Autodesk Fusion 360 part; units mm, degrees
sketch "Sketch2" plane through (0, 0, 0) normal (0, 1, 0) x (1, 0, 0)
  line L0 (76.2, 108.5) -> (-76.2, 108.5)
  line L1 (-76.2, 108.5) -> (-76.2, -108.5)
  line L2 (-76.2, -108.5) -> (76.2, -108.5)
  line L3 (76.2, -108.5) -> (76.2, 108.5)
  line L4 (76.2, 108.5) -> (-76.2, -108.5) construction
  line L5 (-76.2, 108.5) -> (76.2, -108.5) construction
  dimension "d14" = 152.4
  dimension "d15" = 217
extrude "Extrude1" add sketch "Sketch2" against normal blind 3
sketch "Sketch1" plane through (0, 0, 0) normal (0, 1, 0) x (1, 0, 0)
  line L0 (-73.2, -108.5) -> (-76.2, -108.5)
  line L1 (-76.2, -108.5) -> (-76.2, 108.5)
  line L2 (-76.2, 108.5) -> (-73.2, 108.5)
  line L3 (-73.2, 108.5) -> (-73.2, -108.5)
  line L4 (-73.2, -108.5) -> (-76.2, 108.5) construction
  line L5 (-76.2, -108.5) -> (-73.2, 108.5) construction
  line L6 (0, 0) -> (195.5563, 0) construction
  line L7 (73.2, 108.5) -> (76.2, 108.5)
  line L8 (76.2, 108.5) -> (76.2, -108.5)
  line L9 (76.2, -108.5) -> (73.2, -108.5)
  line L10 (73.2, -108.5) -> (73.2, 108.5)
  line L11 (-73.2, 108.5) -> (73.2, 108.5)
  line L12 (73.2, 108.5) -> (73.2, 105.5)
  line L13 (73.2, 105.5) -> (-73.2, 105.5)
  line L14 (-73.2, 105.5) -> (-73.2, 108.5)
  line L15 (73.2, 81.7222) -> (-73.2, 81.7222)
  line L16 (-73.2, 84.7222) -> (73.2, 84.7222)
  line L17 (73.2, 57.9444) -> (-73.2, 57.9444)
  line L18 (-73.2, 60.9444) -> (73.2, 60.9444)
  line L19 (73.2, 34.1667) -> (-73.2, 34.1667)
  line L20 (-73.2, 37.1667) -> (73.2, 37.1667)
  line L21 (73.2, 10.3889) -> (-73.2, 10.3889)
  line L22 (-73.2, 13.3889) -> (73.2, 13.3889)
  line L23 (73.2, -13.3889) -> (-73.2, -13.3889)
  line L24 (-73.2, -10.3889) -> (73.2, -10.3889)
  line L25 (73.2, -37.1667) -> (-73.2, -37.1667)
  line L26 (-73.2, -34.1667) -> (73.2, -34.1667)
  line L27 (73.2, -60.9444) -> (-73.2, -60.9444)
  line L28 (-73.2, -57.9444) -> (73.2, -57.9444)
  line L29 (73.2, -84.7222) -> (-73.2, -84.7222)
  line L30 (-73.2, -81.7222) -> (73.2, -81.7222)
  line L31 (73.2, -108.5) -> (-73.2, -108.5)
  line L32 (-73.2, -105.5) -> (73.2, -105.5)
  point P0 (-74.7, 0)
  dimension "d1" = 217
  dimension "d6" = 3
  dimension "d8" = 152.4
  dimension "d9" = 3
  dimension "d12" = 0
  dimension "d21" = 76.2
extrude "Extrude2" add sketch "Sketch1" along normal blind 42 contours L0 L1 L2 L3 L14 | L7 L8 L9 L10 L12 | L3 L10 L29 L30 | L3 L10 L27 L28 | L3 L10 L15 L16 | L3 L10 L25 L26 | L3 L10 L17 L18 | L3 L10 L23 L24 | L3 L10 L19 L20 | L3 L10 L21 L22
extrude "Extrude3" add sketch "Sketch1" along normal blind 45 contours L3 L10 L31 L32 | L3 L10 L11 L12 L13 L14
chamfer "Chamfer1" distance 1 angle 45 4 edges at (0, -3, -108.5) (-76.2, -3, 0) (76.2, -3, 0) (0, -3, 108.5) measured on face at (-25.4, -3, -36.1667) measured on face at (-25.4, -3, -36.1667) measured on face at (-25.4, -3, -36.1667) measured on face at (-25.4, -3, -36.1667)
equation "d1 = Length"
equation "Length = 217 mm"
equation "Width = 6 in"
equation "Wall_Thickness = 3 mm"
equation "d6 = Wall_Thickness"
equation "d8 = Width"
equation "d9 = Wall_Thickness"
equation "d14 = Width"
equation "d15 = Length"
equation "Height = 45 mm"
equation "d19 = Height - Wall_Thickness"
equation "d21 = Width / 2"
equation "BaseWallThickness_1 = 3 mm"
equation "BearingHolderHeight_1 = 20 mm"
equation "BearingHolderDistance_1 = 80 mm"
equation "BearingHolderDiameter_1 = 7.8 mm"
equation "BaseInsideWidth_1 = 70 mm"
equation "BaseLength_1 = 190 mm"
equation "BaseWallHeight_1 = 100 mm"
equation "d22 = Height"
equation "BaseWallThickness_2 = 3 mm"
equation "BearingHolderHeight_2 = 20 mm"
equation "BearingHolderDistance_2 = 80 mm"
equation "BearingHolderDiameter_2 = 7.8 mm"
equation "BaseInsideWidth_2 = 70 mm"
equation "BaseLength_2 = 190 mm"
equation "BaseWallHeight_2 = 100 mm"
Here's how the part is built. I have some questions about the finished solid (model axes, mm). Coordinates: 2 decimals unless noted, no trailing zeros. Loops run counter-clockwise (first coordinate to the right, second up) from the corner with the lowest first, then second, coordinate; pieces in that order, holes last. Notation, with made-up numbers: (-12, -7) - (7, -7) arc R10 cw to (7, 2) - close; hole circle Ø5 at (81.5, -1.5). An arc over 180 degrees is marked (long way). Answer as CSV lines item,"result".
Q1. If I drill on L1, parallel to X at y = 28, z = 69.5; L2, parallel to Y at x = -19, z = -26; L3, parallel to Y at x = -51.5, z = -36.5, over which ranges is the centre line in solid material (lowest first)? Write a range as [from, to].
Response:
L1,"[-76.2, -73.2], [73.2, 76.2]"
L2,"[-3, 0]"
L3,"[-3, 42]"
Q2. If we section it at A-A, the plane z = -40: Write out the boundary of the cut face in (x, y).
Response:
outline,"(-76.2, -2) - (-75.2, -3) - (75.2, -3) - (76.2, -2) - (76.2, 42) - (73.2, 42) - (73.2, 0) - (-73.2, 0) - (-73.2, 42) - (-76.2, 42) - close"
Q3. We'd pull the mould along Z, two halves only. Please class faces 1 (the face through (-73.2, 21, -71)), 2 (the face through (1, 21, 84.722)): pulls with the +Z half, pulls with the -Z half, needs draft (parallel to the pull), parting line crosses it, or undercut.
Response:
face 1,"undercut"
face 2,"undercut"
Q4. If we section it at B-B, the plane y = 9: Give the number of separate pieces and of enclosed holes in the cut face, and give its area (3 significant figures).
Response:
separate pieces,"1"
enclosed holes,"9"
area,"5,690 mm2"
Q5. For pin 1 (6 mm diameter, centred on x = 12.5, z = -27.5, fed in from +Y), with a flat end and sliding along its axis, tell me the tip position at first contact or that it passes through.
Response:
pin 1,"y = 0"
